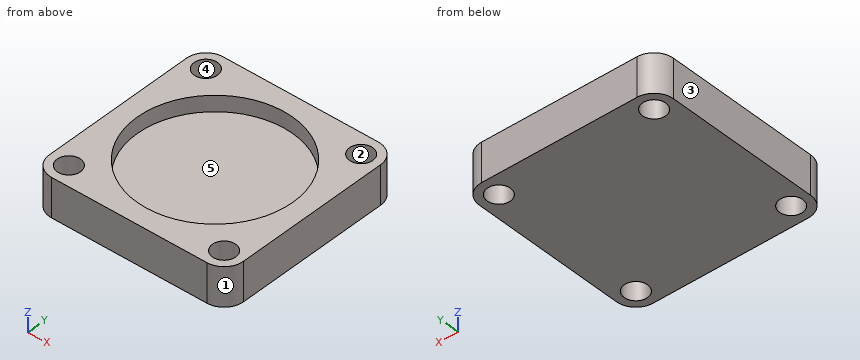
from build123d import *

# Parameters (mm, degrees)
ESQUISSE1_R             = 1.5
BOSS_EXTRU_1_DEPTH      = 5
ESQUISSE2_R             = 10.015
ENL_V_MAT_EXTRU_1_DEPTH = 2.03


with BuildPart() as part:
    # Esquisse1 → Boss.-Extru.1 (new body)
    with BuildSketch(Plane.XY):
        with BuildLine():
            Line((-10, 12.5), (10, 12.5))
            ThreePointArc((10, 12.5), (11.767766953, 11.767766953), (12.5, 10))
            Line((12.5, 10), (12.5, -10))
            ThreePointArc((12.5, -10), (11.767766953, -11.767766953), (10, -12.5))
            Line((10, -12.5), (-10, -12.5))
            ThreePointArc((-10, -12.5), (-11.767766953, -11.767766953), (-12.5, -10))
            Line((-12.5, -10), (-12.5, 10))
            ThreePointArc((-12.5, 10), (-11.767766953, 11.767766953), (-10, 12.5))
        make_face()
        with Locations((-10, 10)):
            Circle(ESQUISSE1_R, mode=Mode.SUBTRACT)
        with Locations((10, 10)):
            Circle(ESQUISSE1_R, mode=Mode.SUBTRACT)
        with Locations((10, -10)):
            Circle(ESQUISSE1_R, mode=Mode.SUBTRACT)
        with Locations((-10, -10)):
            Circle(ESQUISSE1_R, mode=Mode.SUBTRACT)
    extrude(amount=BOSS_EXTRU_1_DEPTH)

    # Esquisse2 → Enlèv. mat.-Extru.1 (cut)
    with BuildSketch(Plane.XY.offset(5)):
        Circle(ESQUISSE2_R)
    extrude(amount=-ENL_V_MAT_EXTRU_1_DEPTH, mode=Mode.SUBTRACT)


solid = part.part
Check sheet for the modelled part. Datum: model origin and axes. Units: mm. Face numbers are marked on the shaded views. A direction names the side the tool comes from. Give positions to 0.01 mm unless a question says otherwise; leave off trailing zeros. Loops run counter-clockwise (first coordinate to the right, second up) from the corner with the lowest first, then second, coordinate; pieces in that order, holes last. Notation, with made-up numbers: M 21.5,28 L 73.5,28 A23 cw 73.5,66 Z; hole C -0.75,51.5 d5. An arc over 180 degrees is marked long. Use a Markdown table: item, result. Add a question column.
Q1. Go/stop test with flat-tipped pins: pin 1 (3 mm diameter, centred on x = 1, y = 9, fed in from +Z); pin 2 (1 mm diameter, centred on x = 2.5, y = 2.5, fed in from +Z). Record where each tip stops, or that it passes through.
Q2. Scan lines: line 1 along Y through (x, z) = (-10, 1.6); line 2 along Y through (x, z) = (0, 3.65) (3 decimals); line 3 along Z through (x, y) = (-8.25, -0.75). Record each from-to range of solid material in increasing order. Write a range as [from, to].
Q3. Sectioned sample at D-D, the plane x = -9. Record the cut outline in (y, z).
Q4. Tool access check on the marked faces 4 and 5. Record the directions out of +Z, -Z, +X, -X, +Y, -Y that give a thin tool (end or side, any length) a straight path to the whole face; none if there is none.
Q5. Mould release check, pull along Y, two halves, no side actions. Record for the marked faces 1, 2 and 3: pulls with the +Y half, pulls with the -Y half, needs draft (parallel to the pull), parting line crosses it, or undercut.
Q6. Sectioned sample at C-C, the plane x = 0. Record the cut outline in (y, z) (3 decimals), then the cut area to 3 significant figures.
Q7. Sectioned sample at A-A, the plane z = 3.45. Record the cut outline in (x, y) (3 decimals).
Q8. Sectioned sample at B-B, the plane z = 0.5. Record the cut outline in (x, y).
Verdict:
| question | item | result |
|---|---|---|
| 1 | pin 1 | z = 5 |
| 1 | pin 2 | z = 2.97 |
| 2 | line 1 | [-12.5, -11.5], [-8.5, 8.5], [11.5, 12.5] |
| 2 | line 2 | [-12.5, -10.015], [10.015, 12.5] |
| 2 | line 3 | [0, 2.97] |
| 3 | outline | M -12.5,0 L -11.12,0 L -11.12,5 L -12.5,5 Z; M -8.88,0 L 8.88,0 L 8.88,5 L 4.39,5 L 4.39,2.97 L -4.39,2.97 L -4.39,5 L -8.88,5 Z; M 11.12,0 L 12.5,0 L 12.5,5 L 11.12,5 Z |
| 4 | face 4 | +Z, -Z |
| 4 | face 5 | +Z |
| 5 | face 1 | pulls with the -Y half |
| 5 | face 2 | undercut |
| 5 | face 3 | needs draft |
| 6 | outline | M -12.5,0 L 12.5,0 L 12.5,5 L 10.015,5 L 10.015,2.97 L -10.015,2.97 L -10.015,5 L -12.5,5 Z |
| 6 | area | 84.3 mm^2 |
| 7 | outline | M -12.5,-10 A2.5 ccw -10,-12.5 L 10,-12.5 A2.5 ccw 12.5,-10 L 12.5,10 A2.5 ccw 10,12.5 L -10,12.5 A2.5 ccw -12.5,10 Z; hole C -10,-10 d3; hole C -10,10 d3; hole C 0,0 d20.03; hole C 10,-10 d3; hole C 10,10 d3 |
| 8 | outline | M -12.5,-10 A2.5 ccw -10,-12.5 L 10,-12.5 A2.5 ccw 12.5,-10 L 12.5,10 A2.5 ccw 10,12.5 L -10,12.5 A2.5 ccw -12.5,10 Z; hole C -10,-10 d3; hole C -10,10 d3; hole C 10,-10 d3; hole C 10,10 d3 |
